For this review, take the finished solid that the model builds, in its own axes (mm). A direction names the side the tool comes from. Give positions to 0.01 mm unless a question says otherwise; leave off trailing zeros. Loops run counter-clockwise (first coordinate to the right, second up) from the corner with the lowest first, then second, coordinate; pieces in that order, holes last.
```python
from build123d import *

# Parameters (mm, degrees)
CUT_EXTRUDE3_DEPTH           = 60
CUT_EXTRUDE5_DEPTH           = 2
CUT_EXTRUDE5_DEPTH_BACK      = 30
SKETCH9_R                    = 38
SKETCH9_R_2                  = 23
SKETCH19_W                   = 12
SKETCH19_H                   = 36.5
CUT_REVOLVE2_ANGLE           = 65
CUT_REVOLVE2_OTHER_WAY_ANGLE = 65
SKETCH21_W                   = 3.25
SKETCH21_H                   = 4
BOSS_EXTRUDE3_DEPTH          = 1.35
CIRPATTERN1_COUNT            = 5
CUT_EXTRUDE9_START           = -5
CUT_EXTRUDE9_DEPTH           = 5
SKETCH23_R                   = 10.5
CUT_EXTRUDE10_DEPTH          = 10
SKETCH24_W                   = 15
SKETCH24_H                   = 8
BOSS_EXTRUDE4_DEPTH          = 8
SKETCH26_W                   = 10
SKETCH26_H                   = 6
CUT_EXTRUDE11_DEPTH          = 10
SKETCH27_W                   = 4
SKETCH27_H                   = 5
CUT_EXTRUDE12_DEPTH          = 5
CUT_EXTRUDE14_DEPTH          = 2
CUT_EXTRUDE14_DEPTH_BACK     = 30
SKETCH29_R                   = 1
CUT_EXTRUDE15_DEPTH          = 15
FILLET1_R                    = 6
FILLET2_R                    = 8
SKETCH31_W                   = 7
SKETCH31_H                   = 5
BOSS_EXTRUDE7_DEPTH          = 13
SKETCH32_R                   = 1.25
CUT_EXTRUDE16_DEPTH          = 7.5


# Read off the part's stored shape, not the designer's step: Cut-Extrude9
with BuildPart() as part:
    # Sketch1 → Revolve1 (revolve)
    with BuildSketch(Plane.XY, mode=Mode.PRIVATE) as revolve1_sk:
        with BuildLine():
            Line((0, 63.427876097), (32, 63.427876097))
            ThreePointArc((32, 63.427876097), (37.656854249, 61.084730346), (40, 55.427876097))
            Line((40, 55.427876097), (40, 28.846818009))
            ThreePointArc((40, 28.846818009), (38.792081772, 24.082439968), (35.460140376, 20.469057744))
            Line((35.460140376, 20.469057744), (28.539859624, 15.958818353))
            ThreePointArc((28.539859624, 15.958818353), (25.207918228, 12.345436129), (24, 7.581058088))
            Line((24, 7.581058088), (24, 3.25))
            Line((24, 3.25), (24.35, 3))
            Line((24.35, 3), (24.35, 0))
            Line((24.35, 0), (22.5, 0))
            Line((22.5, 0), (22.5, 12.5))
            ThreePointArc((22.5, 12.5), (22.353553391, 12.853553391), (22, 13))
            Line((22, 13), (0, 13))
            Line((0, 13), (0, 63.427876097))
        make_face()
    revolve(revolve1_sk.sketch.rotate(Axis((0, 0, 0), (0, 1, 0)), 90), axis=Axis((0, 0, 0), (0, 1, 0)))

    # Sketch11 → Cut-Extrude3 (cut)
    with BuildSketch(Plane(origin=(0, 13, 0), x_dir=(-1, 0, 0), z_dir=(0, -1, 0))):
        with BuildLine():
            Line((-21, 0), (21, 0))
            ThreePointArc((21, 0), (0, 21), (-21, 0))
        make_face()
    extrude(amount=-CUT_EXTRUDE3_DEPTH, mode=Mode.SUBTRACT)

    # Sketch9 → Cut-Extrude5 (cut, two sides: drawn at the far end of the back side and taken through both)
    with BuildSketch(Plane(origin=(0, 55.427876097, 0), x_dir=(1, 0, 0), z_dir=(0, 1, 0)).offset(-CUT_EXTRUDE5_DEPTH_BACK)):
        with Locations(Location((0, 0, 0), (0, 0, 270))):
            Circle(SKETCH9_R)
        with Locations(Location((0, 0, 0), (0, 0, 270))):
            Circle(SKETCH9_R_2, mode=Mode.SUBTRACT)
    extrude(amount=CUT_EXTRUDE5_DEPTH + CUT_EXTRUDE5_DEPTH_BACK, mode=Mode.SUBTRACT)

    # Sketch19 → Cut-Revolve2 (revolve, cut)
    with BuildSketch(Plane(origin=(0, 0, 0), x_dir=(0, 0, -1), z_dir=(1, 0, 0))):
        with Locations((-41.064715832, 37.177876097)):
            Rectangle(SKETCH19_W, SKETCH19_H)
    revolve(axis=Axis((0, 0, 0), (0, 1, 0)), revolution_arc=CUT_REVOLVE2_ANGLE, mode=Mode.SUBTRACT)

    # Sketch19 → Cut-Revolve2 other way (revolve, cut)
    with BuildSketch(Plane(origin=(0, 0, 0), x_dir=(0, 0, -1), z_dir=(1, 0, 0))):
        with Locations((-41.064715832, 37.177876097)):
            Rectangle(SKETCH19_W, SKETCH19_H)
    revolve(axis=Axis((0, 0, 0), (0, -1, 0)), revolution_arc=CUT_REVOLVE2_OTHER_WAY_ANGLE, mode=Mode.SUBTRACT)

    # Sketch21 → Boss-Extrude3 (add)
    with BuildSketch(Plane(origin=(0, 0, 22.5), x_dir=(-1, 0, 0), z_dir=(0, 0, -1))):
        with Locations((0, 2)):
            Rectangle(SKETCH21_W, SKETCH21_H)
    boss_extrude3 = extrude(amount=BOSS_EXTRUDE3_DEPTH)

    # CirPattern1: Boss-Extrude3 ×5 about axis
    cirpattern1_axis = Axis((0, 0, 0), (0, 1, 0))
    for i in range(1, CIRPATTERN1_COUNT):
        add(boss_extrude3.rotate(cirpattern1_axis, i * 360 / CIRPATTERN1_COUNT))

    # Cut-Extrude9 outline → Cut-Extrude9 (cut)
    with BuildSketch(Plane(origin=(0, 63.427876097, 0), x_dir=(1, 0, 0), z_dir=(0, 1, 0)).offset(CUT_EXTRUDE9_START)):
        with BuildLine():
            ThreePointArc((40, 0), (0, 40), (-40, 0))
            Line((-40, 0), (-21, 0))
            ThreePointArc((-21, 0), (0, 21), (21, 0))
            Line((21, 0), (40, 0))
        make_face()
    extrude(amount=CUT_EXTRUDE9_DEPTH, mode=Mode.SUBTRACT)

    # Sketch23 → Cut-Extrude10 (cut)
    with BuildSketch(Plane(origin=(0, 0, -40), x_dir=(-1, 0, 0), z_dir=(0, 0, -1))):
        with Locations((0, 42.137876097)):
            Circle(SKETCH23_R)
    extrude(amount=-CUT_EXTRUDE10_DEPTH, mode=Mode.SUBTRACT)

    # Sketch24 → Boss-Extrude4 (add)
    with BuildSketch(Plane(origin=(0, 58.427876097, 0), x_dir=(1, 0, 0), z_dir=(0, 1, 0))):
        with Locations((0, 30)):
            Rectangle(SKETCH24_W, SKETCH24_H)
    extrude(amount=-BOSS_EXTRUDE4_DEPTH)

    # Sketch26 → Cut-Extrude11 (cut)
    with BuildSketch(Plane(origin=(0, 58.427876097, 0), x_dir=(1, 0, 0), z_dir=(0, 1, 0))):
        with Locations((0, 30)):
            Rectangle(SKETCH26_W, SKETCH26_H)
    extrude(amount=-CUT_EXTRUDE11_DEPTH, mode=Mode.SUBTRACT)

    # Sketch27 → Cut-Extrude12 (cut)
    with BuildSketch(Plane(origin=(7.5, 0, 0), x_dir=(0, 0, -1), z_dir=(1, 0, 0))):
        with Locations((30, 53.927876097)):
            Rectangle(SKETCH27_W, SKETCH27_H)
    extrude(amount=-CUT_EXTRUDE12_DEPTH, mode=Mode.SUBTRACT)

    # Sketch28 → Cut-Extrude14 (cut, two sides: drawn at the far end of the back side and taken through both)
    with BuildSketch(Plane(origin=(0, 55.427876097, 0), x_dir=(1, 0, 0), z_dir=(0, 1, 0)).offset(-CUT_EXTRUDE14_DEPTH_BACK)):
        with BuildLine():
            Line((-22.912878475, -2), (22.912878475, -2))
            ThreePointArc((22.912878475, -2), (0, -23), (-22.912878475, -2))
        make_face()
    extrude(amount=CUT_EXTRUDE14_DEPTH + CUT_EXTRUDE14_DEPTH_BACK, mode=Mode.SUBTRACT)

    # Sketch29 → Cut-Extrude15 (cut)
    with BuildSketch(Plane(origin=(0, 0, 0), x_dir=(-1, 0, 0), z_dir=(0, 0, -1))):
        with Locations((-30.416198487, 60.927876097)):
            Circle(SKETCH29_R)
        with Locations((30.416198487, 60.927876097)):
            Circle(SKETCH29_R)
        with Locations((0, 60.927876097)):
            Circle(SKETCH29_R)
    extrude(amount=-CUT_EXTRUDE15_DEPTH, mode=Mode.SUBTRACT)

    # Fillet1
    fillet1_edges = [part.edges().sort_by_distance(p)[0] for p in [
        (21, 35.713938048, 0),
        (-21, 35.713938048, 0),
    ]]
    fillet(fillet1_edges, radius=FILLET1_R)

    # Fillet2
    fillet2_edges = [part.edges().sort_by_distance(p)[0] for p in [
        (-22.912878475, 41.427876097, 2),
        (22.912878475, 41.427876097, 2),
    ]]
    fillet(fillet2_edges, radius=FILLET2_R)

    # Sketch31 → Boss-Extrude7 (add)
    with BuildSketch(Plane(origin=(0, 58.427876097, 0), x_dir=(1, 0, 0), z_dir=(0, 1, 0))):
        with Locations((0, -29.5)):
            Rectangle(SKETCH31_W, SKETCH31_H)
    extrude(amount=-BOSS_EXTRUDE7_DEPTH)

    # Sketch32 → Cut-Extrude16 (cut)
    with BuildSketch(Plane(origin=(3.5, 0, 0), x_dir=(0, 0, -1), z_dir=(1, 0, 0))):
        with Locations((-29.5, 48.427876097)):
            Circle(SKETCH32_R)
    extrude(amount=-CUT_EXTRUDE16_DEPTH, mode=Mode.SUBTRACT)


solid = part.part
```
Item 1: Clearance check with flat-ended pins moving along their axes: pin 1 Ø3 at (x, z) = (6.5, -30.5) entering from -Y; pin 2 Ø1.5 at (x, y) = (18, 37) entering from -Z; pin 3 Ø1.5 at (x, y) = (-7, 12.5) entering from +Z. State where each tip first meets the part, or that it passes through.
Answer:
pin 1: stops at y = 16.71
pin 2: stops at z = -36.09
pin 3: stops at z = 24.83
Item 2: For L1, parallel to X at y = 55.5, z = 28; L2, parallel to X at y = 44, z = -18.5; L3, parallel to X at y = 8, z = 0, list the stretches that pass through material, from the lowest coordinate up.
Answer:
L1: x = -28.57 to -25.69, -3.5 to 3.5, 25.69 to 28.57
L2: x = -35.46 to -33.19, -13.67 to -9.94, 9.94 to 13.67, 33.19 to 35.46
L3: x = -24.01 to -22.5, 22.5 to 24.01
Item 3: The part is to be moulded in two halves that separate along Y. For faces 1 (the cylindrical face through (0.56, 22.86, 35.06)), 2 (the flat face through (0, 55.428, 39)), 3 (the flat face through (-21, 4, 7)), say which applies: released by +Y, released by -Y, zero draft, split by the parting line, or undercut.
Answer:
face 1: zero draft
face 2: released by -Y
face 3: undercut
Item 4: Take a section at B-B on y = 22. Give the boundary of the cut face in (x, z).
Answer:
outline: (-33.79, 15.76) arc R37.29 ccw (long way) to (33.79, 15.76) - (31.78, 14.82) arc R35.06 ccw to (-31.78, 14.82) - close; hole (-19.25, -8.4) arc R21 ccw to (19.25, -8.4) arc R6 ccw to (13.75, 0) - (-13.75, 0) arc R6 ccw to start
Item 5: Take a section at A-A on y = 40.5. Give the boundary of the cut face in (x, z).
Answer:
outline: (-36.25, 16.9) arc R40 ccw to (-10.37, -38.63) - (-10.37, -36.56) arc R38 cw to (-34.44, 16.06) - close; (-21.08, -9.2) arc R23 ccw to (21.08, -9.2) arc R8 ccw to (13.75, 2) - (-13.75, 2) arc R8 ccw to start; (10.37, -38.63) arc R40 ccw to (36.25, 16.9) - (34.44, 16.06) arc R38 cw to (10.37, -36.56) - close; hole (-19.25, -8.4) arc R21 ccw to (19.25, -8.4) arc R6 ccw to (13.75, 0) - (-13.75, 0) arc R6 ccw to start
Item 6: Tool access review of faces 4 (the cylindrical face through (0, 35, -21)), 5 (the flat face through (-1.8, 50.428, -33.6)), 6 (the flat face through (0, 54, -33)), 7 (the cylindrical face through (0.217, 59.952, 7.395)), 8 (the flat face through (35.04, 38.07, 16.34)): name each direction out of +Z, -Z, +X, -X, +Y, -Y from which nothing blocks a thin tool from reaching the whole face with its end or side.
Answer:
face 4: +Y, -Y
face 5: none
face 6: +Y
face 7: -Z
face 8: +Z, -Y
Item 7: Take a section at C-C on z = -2.5. State how many separate pieces and enclosed holes the cut face has, and give its area (3 significant figures).
Answer:
separate pieces: 2
enclosed holes: 2
area: 722 mm2
